CAD build for the part. Positions are in the model's coordinates, mm. A direction names the side the tool comes from. Coordinates: 2 decimals unless noted, no trailing zeros. Write each loop counter-clockwise with the first axis right and the second up, starting at its lowest first coordinate (ties: lowest second). Pieces come first, ordered by that corner, then holes. Notation, with made-up numbers: (75.5, 47) - (132.5, 47) arc R21 cw to (132.5, 64) - close; hole circle Ø3 at (56, 14). An arc over 180 degrees is marked (long way). Answer in a Markdown table with one row per item. Add a question column.
Q1. Band-saw the part on B-B (z = -4). List the corners of the cut face in (x, y).
Q2. Band-saw the part on A-A (x = 1). List the corners of the cut face in (y, z), and give its area (3 significant figures).
Q3. Two-plate mould, pull along X, no slides. Class faces 1 (the flat face through (7.983, 0.986, -8.254)), 2 (the flat face through (-10.354, 0.986, -4.943)), 3 (the flat face through (0.845, 0.986, 11.448)): +X half, -X half, draft (parallel to the pull), parting line (faces both ways), or undercut.
Q4. Drill centre lines: line 1 along X through (y, z) = (1.6, -10.5); line 2 along X through (y, z) = (0.4, 1); line 3 along Z through (x, y) = (-6, 0.95). Where is each one in solid material? Low to high. Write a range as from..to.
Q5. Pin check, flat tips, straight feed: pin 1 (1 mm diameter, centred on y = 0.5, z = 7.5, fed in from +X); pin 2 (1 mm diameter, centred on x = 8.5, y = 1, fed in from +Z). Stop position of each tip, or through.
Q6. Band-saw the part on C-C (x = -5.5). List the corners of the cut face in (y, z).
Q7. 3-axis set-ups, long thin cutter, end or side, ignore diameter. For faces 4 (the flat face through (-4.764, 0.986, 10.437)), 5 (the flat face through (0.81, 0.99, -11.45)), 6 (the flat face through (-11.14, 0.99, -2.79)), 7 (the flat face through (10.354, 0.986, 4.943)): which of +Z, -Z, +X, -X, +Y, -Y reach the whole face in a straight line?
Autodesk Inventor part; units mm, degrees
ref_plane "YZ Plane" through (0, 0, 0) normal (1, 0, 0) x (0, 1, 0)
ref_plane "XZ Plane" through (0, 0, 0) normal (0, 1, 0) x (-1, 0, 0)
ref_plane "XY Plane" through (0, 0, 0) normal (0, 0, 1) x (1, 0, 0)
sketch "Szkic1" plane through (0, 0, 0) normal (0, 1, 0) x (-1, 0, 0)
  line L0 (0, 12.8914) -> (0, 13)
  line L1 (4.409, 12.114) -> (4.4461, 12.216)
  line L2 (0, 0) -> (13, 0) construction
  line L3 (0, 0) -> (13, 0) construction
  line L4 (12.8025, -2.2574) -> (12.7826, -2.312)
  line L5 (0, -13) -> (0.0571, -12.9898)
  line L6 (0, 13) -> (-1.7143, 9.8513)
  line L7 (-4.506, 12.1936) -> (-1.7143, 9.8513)
  line L8 (-4.506, 12.1936) -> (-5.0309, 8.6423)
  line L9 (-5.0309, 8.6423) -> (-8.3572, 9.9584)
  line L10 (-8.3572, 9.9584) -> (-7.5993, 6.5)
  line L11 (-11.2583, 6.5) -> (-7.5993, 6.5)
  line L12 (-12.8025, 2.2574) -> (-9.4249, 3.3421)
  line L13 (-11.2583, 6.5) -> (-9.4249, 3.3421)
  line L14 (-12.8025, 2.2574) -> (-10, -0.0042)
  line L15 (-12.8025, -2.2574) -> (-10, -0.0042)
  line L16 (-4.4461, -12.216) -> (-1.6431, -9.864)
  line L17 (0, -13) -> (-1.6431, -9.864)
  line L18 (4.5054, -12.1944) -> (1.8242, -9.8405)
  line L19 (1.8242, -9.8405) -> (0, -13)
  line L20 (-8.3562, -9.9586) -> (-5.0917, -8.6067)
  line L21 (-4.4461, -12.216) -> (-5.0917, -8.6067)
  line L22 (-8.3562, -9.9586) -> (-7.5993, -6.5)
  line L23 (-11.2583, -6.5) -> (-7.5993, -6.5)
  line L24 (-11.2583, -6.5) -> (-9.4288, -3.3312)
  line L25 (-12.8025, -2.2574) -> (-9.4288, -3.3312)
  line L26 (4.5054, -12.1944) -> (4.9903, -8.6659)
  line L27 (8.3572, -9.9584) -> (4.9903, -8.6659)
  line L28 (8.3572, -9.9584) -> (7.7142, -6.364)
  line L29 (11.2583, -6.5) -> (7.7142, -6.364)
  line L30 (11.2583, -6.5) -> (9.425, -3.3422)
  line L31 (12.8025, -2.2574) -> (9.425, -3.3422)
  line L32 (0, 13) -> (1.6431, 9.864)
  line L33 (1.6431, 9.864) -> (4.4461, 12.216)
  line L34 (4.4461, 12.216) -> (5.0917, 8.6067)
  line L35 (8.3562, 9.9586) -> (5.0917, 8.6067)
  line L36 (8.3562, 9.9586) -> (7.8406, 6.2068)
  line L37 (11.2583, 6.5) -> (7.8406, 6.2068)
  line L38 (12.8025, 2.2574) -> (9.4288, 3.3312)
  line L39 (11.2583, 6.5) -> (9.4288, 3.3312)
  line L40 (12.8025, -2.2574) -> (10, 0)
  line L41 (12.8025, 2.2574) -> (10, 0)
  line L42 (-0.0571, 12.9898) -> (0, 13)
  arc A0 (5.0917, 8.6067) -> (5.0298, 8.643) centre (0, 0) ccw
  line L43 (-8.4028, 9.904) -> (-8.3572, 9.9584)
  line L44 (8.4028, -9.904) -> (8.3572, -9.9584)
extrude "Wyciągnięcie proste1" add sketch "Szkic1" along normal blind 2
sketch "Szkic2" plane through (0, 2, 0) normal (0, 1, 0) x (1, 0, 0)
  circle A0 centre (0, 0) radius 1.5
  dimension "d9" = 3
hole "Otwór1" at (0, 2, 0) direction (0, -1, 0) diameter 3 depth 8 tip angle 118
properties part number "zebatka" material "Stal"
Checked values:
| question | item | result |
|---|---|---|
| 1 | outline | (-9.81, 0) - (9.81, 0) - (9.81, 2) - (-9.81, 2) - close |
| 2 | outline | (0, -11.09) - (2, -11.09) - (2, -1.12) - (0, -1.12) - close; (0, 1.12) - (2, 1.12) - (2, 11.16) - (0, 11.16) - close |
| 2 | area | 40.0 mm² |
| 3 | face 1 | +X half |
| 3 | face 2 | -X half |
| 3 | face 3 | undercut |
| 4 | line 1 | x = -4.74..-2.58, -1.44..1.31, 2.4..4.75 |
| 4 | line 2 | x = -11.24..-1.12, 1.12..11.24 |
| 4 | line 3 | z = -9.05..8.98 |
| 5 | pin 1 | stops at x = 7.93 |
| 5 | pin 2 | stops at z = 9.96 |
| 6 | outline | (0, -8.86) - (2, -8.86) - (2, 8.78) - (0, 8.78) - close |
| 7 | face 4 | +Z, +Y, -Y |
| 7 | face 5 | -Z, +Y, -Y |
| 7 | face 6 | -X, +Y, -Y |
| 7 | face 7 | +X, +Y, -Y |
